```python
from build123d import *

# Parameters (mm, degrees)
SKETCH001_W  = 20
SKETCH001_H  = 28
PAD001_DEPTH = 2.5
SKETCH002_W  = 20
SKETCH002_H  = 5
PAD002_DEPTH = 23
POCKET_DEPTH = 5
SKETCH004_W  = 2.855627
SKETCH004_H  = 23
PAD003_DEPTH = 23


with BuildPart() as part:
    # Sketch001 → Pad001 (new body, symmetric)
    with BuildSketch(Plane.XZ):
        Rectangle(SKETCH001_W, SKETCH001_H)
        with BuildLine():
            ThreePointArc((3.25, 2.625), (0, 5.875), (-3.25, 2.625))
            Line((-3.25, 2.625), (-3.25, -2.625))
            ThreePointArc((-3.25, -2.625), (0, -5.875), (3.25, -2.625))
            Line((3.25, 2.625), (3.25, -2.625))
        make_face(mode=Mode.SUBTRACT)
    extrude(amount=PAD001_DEPTH, both=True)

    # Sketch002 (on Face10 of Pad001) → Pad002 (join)
    with BuildSketch(Plane.XZ.offset(2.5)):
        with Locations((0, -11.5)):
            Rectangle(SKETCH002_W, SKETCH002_H)
    extrude(amount=PAD002_DEPTH)

    # Sketch003 (on Face13 of Pad002) → Pocket (cut)
    with BuildSketch(Plane(origin=(0, 0, -9), x_dir=(-1, 0, 0), z_dir=(0, 0, 1))):
        with BuildLine():
            ThreePointArc((3.25, 14.125), (0, 17.375), (-3.25, 14.125))
            Line((-3.25, 14.125), (-3.25, 8.875))
            ThreePointArc((-3.25, 8.875), (0, 5.625), (3.25, 8.875))
            Line((3.25, 14.125), (3.25, 8.875))
        make_face()
    extrude(amount=-POCKET_DEPTH, mode=Mode.SUBTRACT)

    # Sketch004 (on Face5 of Pocket) → Pad003 (join)
    with BuildSketch(Plane.XZ.offset(2.5)):
        with Locations((-8.5721865, 2.5)):
            Rectangle(SKETCH004_W, SKETCH004_H)
        with Locations((8.5721865, 2.5)):
            Rectangle(SKETCH004_W, SKETCH004_H)
    extrude(amount=PAD003_DEPTH)


solid = part.part
```
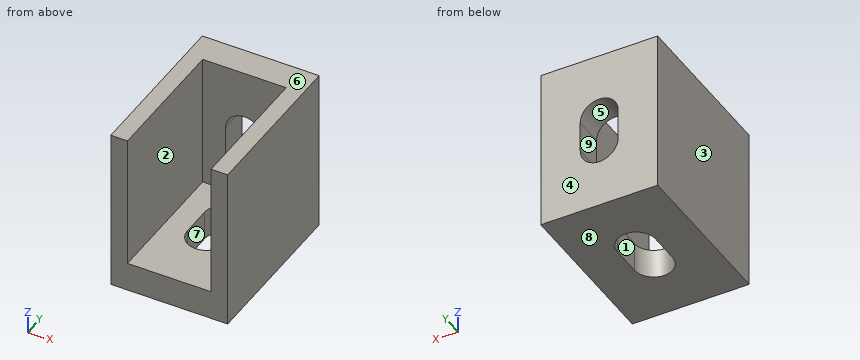
Design review of the part built by this model. Coordinates are the model's own, in mm. Face numbers are marked on the shaded views. A direction names the side the tool comes from. Coordinates: 2 decimals unless noted, no trailing zeros. Loops run counter-clockwise (first coordinate to the right, second up) from the corner with the lowest first, then second, coordinate; pieces in that order, holes last.
Q1. We need section A-A on x = 0. State the section outline as (y, z) points (3 decimals), and give its area (4 significant figures).
Reported:
outline: (-25.5, -14) - (-17.375, -14) - (-17.375, -9) - (-25.5, -9) - close; (-5.625, -14) - (2.5, -14) - (2.5, -5.875) - (-2.5, -5.875) - (-2.5, -9) - (-5.625, -9) - close; (-2.5, 5.875) - (2.5, 5.875) - (2.5, 14) - (-2.5, 14) - close
area: 137.5 mm2
Q2. To check wall thickness, follow line 1 (X direction, y = -22.75, z = -4.75); line 2 (Z direction, x = -3.5, y = -15); line 3 (Y direction, x = -3.25, z = 11.5). State the ranges of each line that lie inside material, in increasing order.
Reported:
line 1: x = -10 to -7.14, 7.14 to 10
line 2: z = -14 to -9
line 3: y = -2.5 to 2.5
Q3. We need section C-C on y = -23.5. State the section outline as (x, z) points, and give its area (3 significant figures).
Reported:
outline: (-10, -14) - (10, -14) - (10, 14) - (7.14, 14) - (7.14, -9) - (-7.14, -9) - (-7.14, 14) - (-10, 14) - close
area: 231 mm2
Q4. For pin 1 (10 mm diameter, centred on x = 4, z = 4.5, fed in from -Y); pin 2 (11.5 mm diameter, centred on x = 0, y = -13.5, fed in from +Z), all flat-tipped, find the tip position at first contact; note any pin that passes through.
Reported:
pin 1: stops at y = -25.5
pin 2: stops at z = -9
Q5. Tool access review of the marked faces 1, 2, 3, 4 and 5: name each direction out of +Z, -Z, +X, -X, +Y, -Y from which nothing blocks a thin tool from reaching the whole face with its end or side.
Reported:
face 1: +Z, -Z
face 2: +Z, -Y
face 3: +Z, -Z, -X, +Y, -Y
face 4: +Z, -Z, +X, -X, +Y
face 5: +Y, -Y
Q6. The part is to be moulded in two halves that separate along Z. For the marked faces 6, 7, 8 and 9, say which applies: +Z half, -Z half, draft (parallel to the pull), parting line (faces both ways), or undercut.
Reported:
face 6: +Z half
face 7: draft
face 8: -Z half
face 9: undercut
Q7. We need section B-B on z = 11.5. State the section outline as (x, y) points, and give its area (3 significant figures).
Reported:
outline: (-10, -25.5) - (-7.14, -25.5) - (-7.14, -2.5) - (7.14, -2.5) - (7.14, -25.5) - (10, -25.5) - (10, 2.5) - (-10, 2.5) - close
area: 231 mm2
Q8. We need section D-D on x = 5.75. State the section outline as (y, z) points, and give its area (3 significant figures).
Reported:
outline: (-25.5, -14) - (2.5, -14) - (2.5, 14) - (-2.5, 14) - (-2.5, -9) - (-25.5, -9) - close
area: 255 mm2
